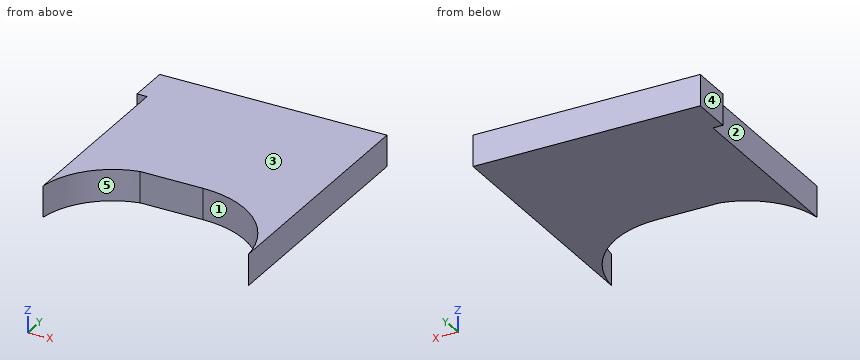
```python
from build123d import *

# Parameters (mm, degrees)
BOSS_EXTRUDE3_DEPTH = 3.175


with BuildPart() as part:
    # Sketch3 → Boss-Extrude3 (new body)
    with BuildSketch(Plane.XY):
        with BuildLine():
            Line((30.293540828, -9.162699553), (26.82456956, -9.162699553))
            Line((26.82456956, -9.162699553), (23.910273162, -9.162699553))
            ThreePointArc((23.910273162, -9.162699553), (19.744450184, -11.435363695), (17.679624466, -15.708018391))
            Line((17.679624466, -15.708018391), (17.679624466, 3.279335675))
            Line((17.679624466, 3.279335675), (16.66456956, 3.279335675))
            Line((16.66456956, 3.279335675), (16.66456956, 7.406835675))
            Line((16.66456956, 7.406835675), (38.515978397, 7.406835675))
            Line((38.515978397, 7.406835675), (39.783204201, 7.406835675))
            Line((39.783204201, 7.406835675), (39.783204201, -6.622699553))
            Line((39.783204201, -6.622699553), (39.783204201, -9.162699553))
            Line((39.783204201, -9.162699553), (39.783204201, -17.86799591))
            ThreePointArc((39.783204201, -17.86799591), (36.732405161, -11.668678888), (30.293540828, -9.162699553))
        make_face()
    extrude(amount=BOSS_EXTRUDE3_DEPTH)


solid = part.part
```
Work out the finished part from the listing and answer in its coordinate system (mm). Face numbers are marked on the shaded views. A direction names the side the tool comes from. Round coordinates to 2 decimals unless told otherwise and drop trailing zeros. Loops run counter-clockwise (first coordinate to the right, second up) from the corner with the lowest first, then second, coordinate; pieces in that order, holes last. Notation, with made-up numbers: M 55.5,4 L 68.5,4 A31 cw 68.5,33 Z; hole C -34.75,81 d6. An arc over 180 degrees is marked long. One line per question, with ' | ' between items.
Q1. The mould has two halves that part along X. Classify the marked faces 1, 2 and 3: +X half, -X half, draft (parallel to the pull), parting line (faces both ways), or undercut.
Conclusion:
face 1: undercut | face 2: -X half | face 3: draft
Q2. Find section C-C, the plane x = 30. Give the vertices of the cut face in (y, z) (3 decimals), then the cut area to 3 significant figures.
Conclusion:
outline: M -9.163,0 L 7.407,0 L 7.407,3.175 L -9.163,3.175 Z | area: 52.6 mm2
Q3. Find section A-A, the plane y = -12.5. Give the vertices of the cut face in (x, z) (3 decimals).
Conclusion:
outline: M 17.68,0 L 18.896,0 L 18.896,3.175 L 17.68,3.175 Z; M 37.535,0 L 39.783,0 L 39.783,3.175 L 37.535,3.175 Z
Q4. Each of these flat-tipped pins is pushed along its axis until it touches: pin 1 Ø1.6 at (x, z) = (26.5, 1.5) entering from -Y; pin 2 Ø0.5 at (x, z) = (17, 2) entering from -Y. Where does it stop, or does it pass through?
Conclusion:
pin 1: stops at y = -9.16 | pin 2: stops at y = 3.28
Q5. Find section B-B, the plane z = 0.45. Give the vertices of the cut face in (x, y) (3 decimals), then the cut area to 3 significant figures.
Conclusion:
outline: M 16.665,3.279 L 17.68,3.279 L 17.68,-15.708 A7.763 cw 23.91,-9.163 L 30.294,-9.163 A9.525 cw 39.783,-17.868 L 39.783,7.407 L 16.665,7.407 Z | area: 401 mm2
Q6. Find section D-D, the plane y = -2. Give the vertices of the cut face in (x, z) (3 decimals).
Conclusion:
outline: M 17.68,0 L 39.783,0 L 39.783,3.175 L 17.68,3.175 Z
Q7. Consider line 1 along Y through (x, z) = (29.25, 1.7); line 2 along X through (y, z) = (-7.75, 0.35); line 3 along X through (y, z) = (-13, 0.75). Determine where each line is inside the solid, lowest interval first. Write a range as from..to.
Conclusion:
line 1: y = -9.16..7.41 | line 2: x = 17.68..39.78 | line 3: x = 17.68..18.59, 37.93..39.78
Q8. A tool of negligible diameter and unlimited length cuts with its end or side. For the marked faces 4 and 5, from which of +Z, -Z, +X, -X, +Y, -Y can it reach the whole face along a straight path? Write none if from no direction.
Conclusion:
face 4: +Z, -Z, -X, +Y, -Y | face 5: +Z, -Z, -Y
